The figure shows three views and two pictorial views of one solid part (mm, origin at its lowest corner). Answer the questions. Coordinates: 2 decimals unless noted, no trailing zeros. Write each loop counter-clockwise with the first axis right and the second up, starting at its lowest first coordinate (ties: lowest second). Pieces come first, ordered by that corner, then holes.
Item 1: Section B-B (y = 120) is taken. Give the vertices of the cut face in (x, z), then the cut area to 3 significant figures.
Item 2: Section D-D (x = 21.5) is taken. Give the vertices of the cut face in (y, z) (1 decimal), then the cut area to 3 significant figures.
Item 3: Each of these flat-tipped pins is pushed along its axis until it touches: P1, Ø3, axis at y = 72.5, z = 4.5, coming from the +X side; P2, Ø6, axis at x = 228.5, z = 3.5, coming from the -Y side; P3, Ø4, axis at y = 236, z = 6, coming from the -X side. Where does it stop, or does it pass through?
Item 4: Straight lines are drawn through the part: probe 1 along Y at (x, z) = (175, 7.25); probe 2 along Y at (x, z) = (163, 7.75); probe 3 along X at (y, z) = (120, 7.5) (1 decimal). For each, find the intervals that lie inside material, in ascending order.
Item 5: Section A-A (x = 175) is taken. Give the vertices of the cut face in (y, z).
Item 6: Section C-C (z = 6) is taken. Give the vertices of the cut face in (x, y).
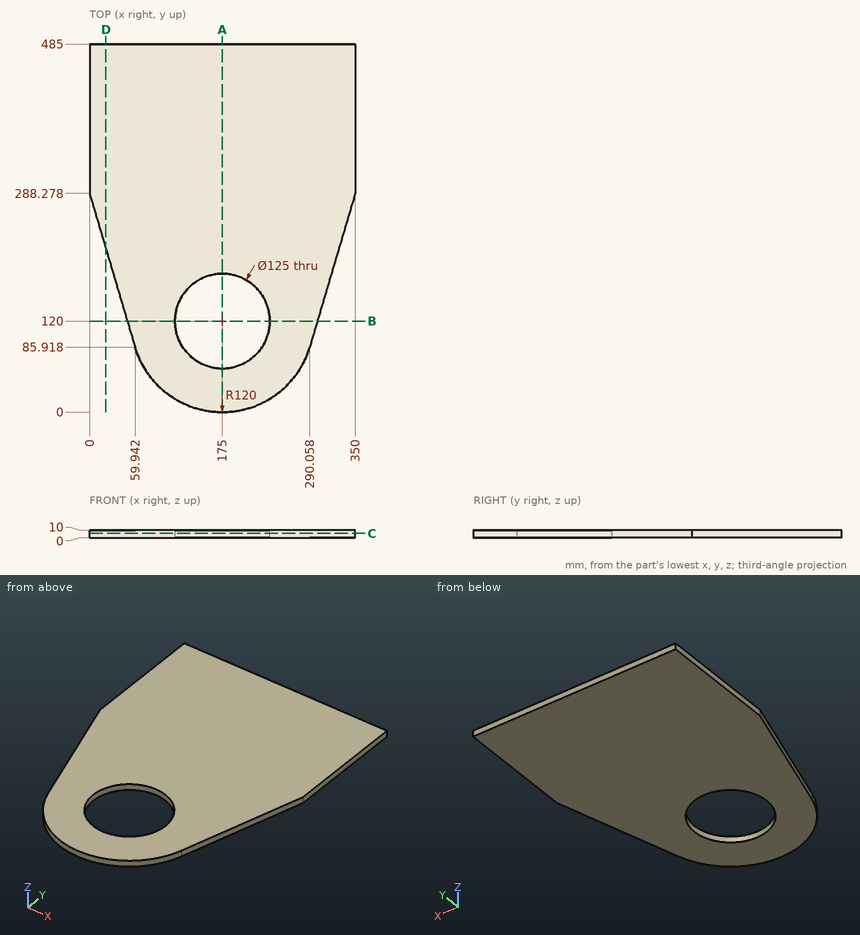
Established:
1. outline: (49.85, 0) - (112.5, 0) - (112.5, 10) - (49.85, 10) - close; (237.5, 0) - (300.15, 0) - (300.15, 10) - (237.5, 10) - close
1. area: 1,250 mm2
2. outline: (215.7, 0) - (485, 0) - (485, 10) - (215.7, 10) - close
2. area: 2,690 mm2
3. P1: stops at x = 285.83
3. P2: stops at y = 11.14
3. P3: stops at x = 14.89
4. probe 1: y = 0 to 57.5, 182.5 to 485
4. probe 2: y = 0.6 to 58.66, 181.34 to 485
4. probe 3: x = 49.8 to 112.5, 237.5 to 300.2
5. outline: (0, 0) - (57.5, 0) - (57.5, 10) - (0, 10) - close; (182.5, 0) - (485, 0) - (485, 10) - (182.5, 10) - close
6. outline: (0, 288.28) - (59.94, 85.92) arc R120 ccw to (290.06, 85.92) - (350, 288.28) - (350, 485) - (0, 485) - close; hole circle Ø125 at (175, 120)
